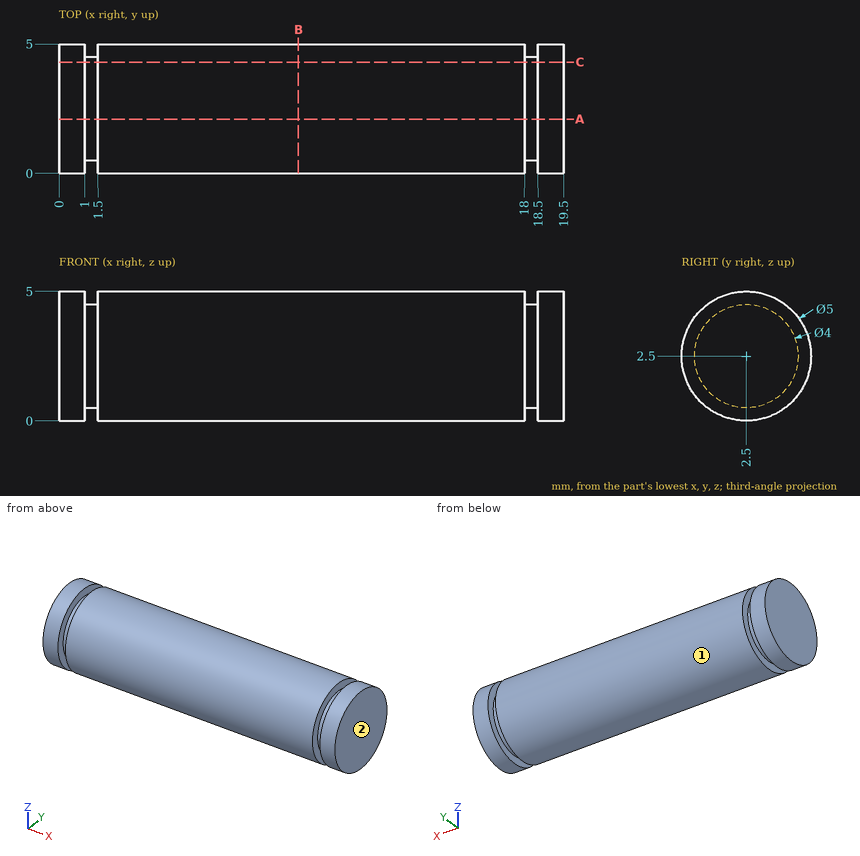
Job drawing, mm, ordinate dimensions from the low corner. One solid piece. Coordinates: 2 decimals unless noted, no trailing zeros. Order: outer loops, then holes, each group sorted by start corner. A loop starts at its lowest first (then second) coordinate and runs counter-clockwise, first axis right, second up. Notation, with made-up numbers: M -8,38 L 0,38 A21 cw 0,77 Z; hole C 23.5,75 d9. An arc over 180 degrees is marked long. Return JSON: item names as keys, results as strings.
1. Saw through at C-C (y = 4.3). Give the cut face in (x, z).
Ans:
{"outline": "M 0,0.77 L 1,0.77 L 1,1.63 L 1.5,1.63 L 1.5,0.77 L 18,0.77 L 18,1.63 L 18.5,1.63 L 18.5,0.77 L 19.5,0.77 L 19.5,4.23 L 18.5,4.23 L 18.5,3.37 L 18,3.37 L 18,4.23 L 1.5,4.23 L 1.5,3.37 L 1,3.37 L 1,4.23 L 0,4.23 Z"}
2. Saw through at B-B (x = 9.25). Give the cut face in (y, z), and give its area (3 significant figures).
Ans:
{"outline": "C 2.5,2.5 d5", "area": "19.6 mm^2"}
3. Flat gauge pins, fed straight in: pin 1 (1 mm diameter, centred on x = 8.5, z = 4, fed in from +Y); pin 2 (3 mm diameter, centred on y = 3, z = 1.5, fed in from -X). Where does each tip first touch, or does it go through?
Ans:
{"pin 1": "y = 4.79", "pin 2": "x = 0"}
4. Saw through at A-A (y = 2.1). Give the cut face in (x, z), and give its area (3 significant figures).
Ans:
{"outline": "M 0,0.03 L 1,0.03 L 1,0.54 L 1.5,0.54 L 1.5,0.03 L 18,0.03 L 18,0.54 L 18.5,0.54 L 18.5,0.03 L 19.5,0.03 L 19.5,4.97 L 18.5,4.97 L 18.5,4.46 L 18,4.46 L 18,4.97 L 1.5,4.97 L 1.5,4.46 L 1,4.46 L 1,4.97 L 0,4.97 Z", "area": "95.2 mm^2"}
5. Pull direction Y, two halves, no side cores. Call the marked faces 1 and 2: +Y half, -Y half, draft (parallel to the pull), parting line (faces both ways), or undercut.
Ans:
{"face 1": "parting line", "face 2": "draft"}
6. Drill centre lines: probe 1 along X at (y, z) = (4.15, 0.8); probe 2 along Z at (x, y) = (16, 1.25); probe 3 along Y at (x, z) = (5.5, 2.4). Where is each one in solid material? Low to high.
Ans:
{"probe 1": "0 to 1, 1.5 to 18, 18.5 to 19.5", "probe 2": "0.33 to 4.67", "probe 3": "0 to 5"}
